Could you check a few things on this model? Use its own coordinates, in mm. Face numbers are marked on the shaded views. A direction names the side the tool comes from. Round coordinates to 2 decimals unless told otherwise and drop trailing zeros. Write each loop counter-clockwise with the first axis right and the second up, starting at its lowest first coordinate (ties: lowest second). Pieces come first, ordered by that corner, then holes. Notation, with made-up numbers: (40, 47) -> (50, 47) arc R10 cw to (50, 52) -> close; hole circle Ø1 at (65.5, 66.25). An arc over 180 degrees is marked (long way). Answer in a Markdown table with one row per item. Add a question column.
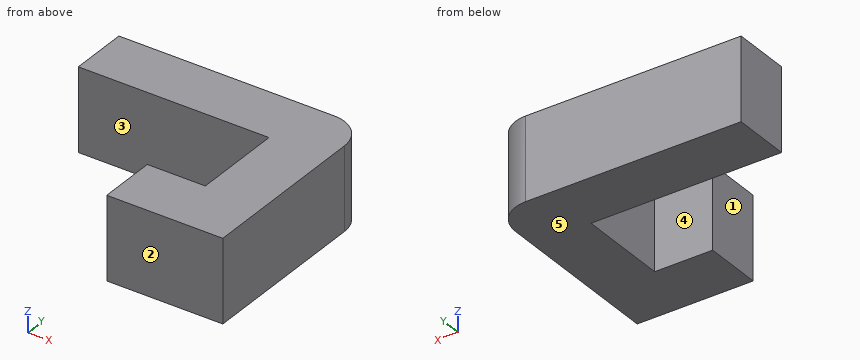
```python
from build123d import *

# Parameters (mm, degrees)
BOX001_W     = 7
BOX001_H     = 25
BOX001_DEPTH = 10
FILLET_R     = 4
BOX_W        = 7
BOX_H        = 7
BOX_DEPTH    = 10
BOX002_W     = 23
BOX002_H     = 7
BOX002_DEPTH = 10


with BuildPart() as fillet_body:
    # Box001 → Box001 (new body)
    with BuildSketch(Plane(origin=(10, 0, 0), x_dir=(1, 0, 0), z_dir=(0, 0, 1))):
        with Locations((3.5, 12.5)):
            Rectangle(BOX001_W, BOX001_H)
    extrude(amount=BOX001_DEPTH)

    # Fillet
    fillet_edges = [fillet_body.edges().sort_by_distance(p)[0] for p in [
        (17, 25, 5),
    ]]
    fillet(fillet_edges, radius=FILLET_R)


with BuildPart() as cubo:
    # Box → Box (new body)
    with BuildSketch(Plane(origin=(3, 0, 0), x_dir=(1, 0, 0), z_dir=(0, 0, 1))):
        with Locations((3.5, 3.5)):
            Rectangle(BOX_W, BOX_H)
    extrude(amount=BOX_DEPTH)


with BuildPart() as fusion:
    # Box002 → Box002 (new body)
    with BuildSketch(Plane(origin=(-13, 18, 0), x_dir=(1, 0, 0), z_dir=(0, 0, 1))):
        with Locations((11.5, 3.5)):
            Rectangle(BOX002_W, BOX002_H)
    extrude(amount=BOX002_DEPTH)

    # Fusion: union Fillet body, Cubo
    add(fillet_body.part)
    add(cubo.part)


solid = fusion.part
```
(1) Suppose I cut it at B-B, the plane z = 3. Please give me the cut outline in (x, y), then the cut area to 3 significant figures.
(2) I need wall thicknesses on L1, parallel to Y at x = 7.75, z = 5.25; L2, parallel to X at y = 15.5, z = 1.25; L3, parallel to Y at x = 1.5, z = 2. Which ranges of each line are inside material? Lowest first, please.
(3) If we mould it in two halves opening along Y, with no side actions, what happens to the marked faces 1, 2 and 3? For each: pulls with the +Y half, pulls with the -Y half, needs draft (parallel to the pull), parting line crosses it, or undercut.
(4) Suppose I cut it at C-C, the plane x = -7. Please give me the cut outline in (y, z).
(5) For P1, Ø5.5, axis at y = 2, z = 4, coming from the -X side; P2, Ø3, axis at y = 14, z = 4.5, coming from the -X side, each with a flat end and sliding along its axis, tell me the tip position at first contact or that it passes through.
(6) Suppose I cut it at A-A, the plane x = 5.75. Please give me the cut outline in (y, z).
(7) On a 3-axis mill with a long thin cutter (end or side, diameter ignored), from which of +Z, -Z, +X, -X, +Y, -Y can I reach the whole of each face in a straight line? I mean the marked faces 4 and 5. Say none if no direction works.
(8) Suppose I cut it at D-D, the plane y = 8.75. Please give me the cut outline in (x, z), then the cut area to 3 significant figures.
Response:
| question | item | result |
|---|---|---|
| 1 | outline | (-13, 18) -> (10, 18) -> (10, 7) -> (3, 7) -> (3, 0) -> (17, 0) -> (17, 21) arc R4 ccw to (13, 25) -> (-13, 25) -> close |
| 1 | area | 382 mm² |
| 2 | L1 | 0 to 7, 18 to 25 |
| 2 | L2 | 10 to 17 |
| 2 | L3 | 18 to 25 |
| 3 | face 1 | needs draft |
| 3 | face 2 | pulls with the -Y half |
| 3 | face 3 | undercut |
| 4 | outline | (18, 0) -> (25, 0) -> (25, 10) -> (18, 10) -> close |
| 5 | P1 | x = 3 |
| 5 | P2 | x = 10 |
| 6 | outline | (0, 0) -> (7, 0) -> (7, 10) -> (0, 10) -> close; (18, 0) -> (25, 0) -> (25, 10) -> (18, 10) -> close |
| 7 | face 4 | +Z, -Z, -X |
| 7 | face 5 | -Z, +X, -X, +Y, -Y |
| 8 | outline | (10, 0) -> (17, 0) -> (17, 10) -> (10, 10) -> close |
| 8 | area | 70.0 mm² |
